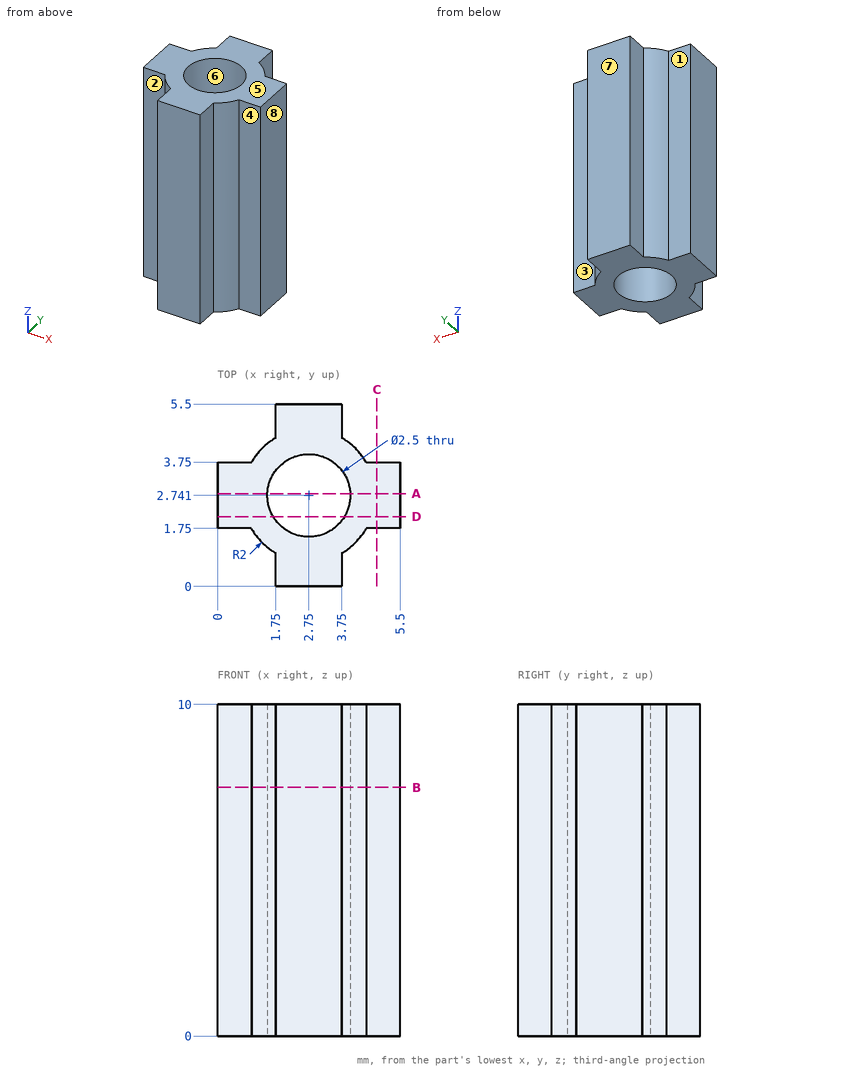
Part print with two shaded views. Sizes in mm from the minimum x, y, z corner. A direction names the side the tool comes from. Coordinates: 2 decimals unless noted, no trailing zeros. Write each loop counter-clockwise with the first axis right and the second up, starting at its lowest first coordinate (ties: lowest second). Pieces come first, ordered by that corner, then holes. Notation, with made-up numbers: (38, -0.5) - (83, -0.5) arc R23 ccw to (83, 38.5) - close; hole circle Ø10 at (48.25, 37.25). An arc over 180 degrees is marked (long way). Put each result on its own line as item: value.
1. Band-saw the part on C-C (x = 4.8). Write the cut outline in (y, z), then the cut area to 3 significant figures.
Final values:
outline: (1.75, 0) - (3.75, 0) - (3.75, 10) - (1.75, 10) - close
area: 20.0 mm²
2. Band-saw the part on B-B (z = 7.5). Write the cut outline in (x, y).
Final values:
outline: (0, 1.75) - (1.01, 1.75) arc R2 ccw to (1.75, 1.01) - (1.75, 0) - (3.75, 0) - (3.75, 1.01) arc R2 ccw to (4.49, 1.75) - (5.5, 1.75) - (5.5, 3.75) - (4.48, 3.75) arc R2 ccw to (3.75, 4.47) - (3.75, 5.5) - (1.75, 5.5) - (1.75, 4.47) arc R2 ccw to (1.02, 3.75) - (0, 3.75) - close; hole circle Ø2.5 at (2.75, 2.74)
3. Two-plate mould, pull along Y, no slides. Class the marked faces 6, 7 and 8: +Y half, -Y half, draft (parallel to the pull), parting line (faces both ways), or undercut.
Final values:
face 6: undercut
face 7: +Y half
face 8: draft
4. 3-axis set-ups, long thin cutter, end or side, ignore diameter. For the marked faces 1, 2, 3, 4 and 5: which of +Z, -Z, +X, -X, +Y, -Y reach the whole face in a straight line?
Final values:
face 1: +Z, -Z, -X, +Y
face 2: +Z, -Z, -X, -Y
face 3: +Z, -Z, +X, +Y
face 4: +Z, -Z, +X, -Y
face 5: +Z, +X, -X, +Y, -Y
5. Flat gauge pins, fed straight in: pin 1 Ø1.5 at (y, z) = (1.5, 6.5) entering from -X; pin 2 Ø1 at (y, z) = (4.5, 2.5) entering from +X; pin 3 Ø0.5 at (y, z) = (0.5, 4) entering from +X; pin 4 Ø0.8 at (y, z) = (0.5, 3.5) entering from -X. Where does each tip first touch, or does it go through?
Final values:
pin 1: stops at x = 0
pin 2: stops at x = 4.3
pin 3: stops at x = 3.75
pin 4: stops at x = 1.75
6. Probe line 1 along Y through (x, z) = (2.75, 3.5); line 2 along Y through (x, z) = (0.85, 5.25); line 3 along Y through (x, z) = (3.3, 1.5). List the from-to ranges inside material, lowest first. Write a range as [from, to].
Final values:
line 1: y = [0, 1.49], [3.99, 5.5]
line 2: y = [1.75, 3.75]
line 3: y = [0, 1.62], [3.86, 5.5]
7. Band-saw the part on A-A (y = 2.8). Write the cut outline in (x, z).
Final values:
outline: (0, 0) - (1.5, 0) - (1.5, 10) - (0, 10) - close; (4, 0) - (5.5, 0) - (5.5, 10) - (4, 10) - close
8. Band-saw the part on D-D (y = 2.1). Write the cut outline in (x, z).
Final values:
outline: (0, 0) - (1.68, 0) - (1.68, 10) - (0, 10) - close; (3.82, 0) - (5.5, 0) - (5.5, 10) - (3.82, 10) - close
